Geometry check sheet. Reference: the model listing, model coordinates, mm. A direction names the side the tool comes from. Round coordinates to 2 decimals unless told otherwise and drop trailing zeros. Write each loop counter-clockwise with the first axis right and the second up, starting at its lowest first coordinate (ties: lowest second). Pieces come first, ordered by that corner, then holes. Notation, with made-up numbers: M 62,9 L 80,9 A13 cw 80,20 Z; hole C 50,9.5 d6. An arc over 180 degrees is marked long. Use a Markdown table: item, result.
```python
from build123d import *


with BuildPart() as f1:
    # F0 (on Front) → F1 (revolve)
    with BuildSketch(Plane.XZ):
        with BuildLine():
            Line((-102.970031, -6.875699), (-102.970031, -21.875699))
            Line((-102.970031, -21.875699), (97.029969, -21.875699))
            Line((97.029969, -21.875699), (97.029969, 48.124301))
            Line((97.029969, 48.124301), (91.029969, 48.124301))
            Line((91.029969, 48.124301), (91.029969, -4.875699))
            ThreePointArc((91.029969, -4.875699), (90.444182, -6.289912), (89.029969, -6.875699))
            Line((89.029969, -6.875699), (87.029969, -6.875699))
            ThreePointArc((87.029969, -6.875699), (85.615755, -6.289912), (85.029969, -4.875699))
            Line((85.029969, -4.875699), (85.029969, 48.124301))
            Line((85.029969, 48.124301), (79.029969, 48.124301))
            Line((79.029969, 48.124301), (79.029969, -4.875699))
            ThreePointArc((79.029969, -4.875699), (78.444182, -6.289912), (77.029969, -6.875699))
            Line((77.029969, -6.875699), (75.029969, -6.875699))
            ThreePointArc((75.029969, -6.875699), (73.615755, -6.289912), (73.029969, -4.875699))
            Line((73.029969, -4.875699), (73.029969, 48.124301))
            Line((73.029969, 48.124301), (67.029969, 48.124301))
            Line((67.029969, 48.124301), (67.029969, -4.875699))
            ThreePointArc((67.029969, -4.875699), (66.444182, -6.289912), (65.029969, -6.875699))
            Line((65.029969, -6.875699), (-102.970031, -6.875699))
        make_face()
    revolve(axis=Axis((-4.417114, 0, -91.875699), (1, 0, 0)))


solid = f1.part
```
Item 1: Cross-section at A-A, the plane x = -33. Record the cut outline in (y, z).
Outcome:
| item | result |
|---|---|
| outline | C 0,-91.88 d170; hole C 0,-91.88 d140 |
Item 2: Go/stop test with flat-tipped pins: pin 1 (2 mm diameter, centred on x = 76.5, y = 27.5, fed in from +Z); pin 2 (2 mm diameter, centred on x = -81.5, y = 58.5, fed in from -Z); pin 3 (12 mm diameter, centred on x = 56, y = -45.5, fed in from +Z). Record where each tip stops, or that it passes through.
Outcome:
| item | result |
|---|---|
| pin 1 | stops at z = -11.11 |
| pin 2 | stops at z = -154.48 |
| pin 3 | stops at z = -16.61 |
Item 3: Mould release check, pull along X, two halves, no side actions. Record for faces 4 (the face through (-102.97, -70, -80)), 5 (the face through (-20.15, -25.53, -10.8)), 6 (the face through (85.03, -64, -152)), 7 (the face through (73.03, -64, -152)): +X half, -X half, draft (parallel to the pull), parting line (faces both ways), or undercut.
Outcome:
| item | result |
|---|---|
| face 4 | -X half |
| face 5 | draft |
| face 6 | undercut |
| face 7 | undercut |
Item 4: Material ranges on line 1 along X through (y, z) = (95, -12); line 2 along Z through (x, y) = (-44, 0); line 3 along Y through (x, z) = (9, -137), recorded low to high. Write a range as from..to.
Outcome:
| item | result |
|---|---|
| line 1 | x = 67.03..73.03, 79.03..85.03, 91.03..97.03 |
| line 2 | z = -176.88..-161.88, -21.88..-6.88 |
| line 3 | y = -72.03..-53.51, 53.51..72.03 |
Item 5: Access from +Z, -Z, +X, -X, +Y, -Y to the whole of each face (thin tool, end or side, straight path). Record for faces 1 (the face through (76.02, -25.53, -10.8)), 2 (the face through (93.988, 85.188, -202.975)), 3 (the face through (67.03, -64, -32)).
Outcome:
| item | result |
|---|---|
| face 1 | none |
| face 2 | +X, -X |
| face 3 | -X |
